Check sheet for the modelled part. Datum: model origin and axes. Units: mm. Face numbers are marked on the shaded views. A direction names the side the tool comes from. Give positions to 0.01 mm unless a question says otherwise; leave off trailing zeros. Order: outer loops, then holes, each group sorted by start corner. A loop starts at its lowest first (then second) coordinate and runs counter-clockwise, first axis right, second up.
```python
from build123d import *

# Parameters (mm, degrees)
F0_R     = 3.175
F1_DEPTH = 19.05
F2_R     = 3.175
F3_DEPTH = 25.4
F4_R     = 6.35


with BuildPart() as f1:
    # F0 (on Top) → F1 (new body)
    with BuildSketch(Plane.XY):
        Polygon((21.1725122346, -375.6896027952), (21.1725122346, -220.1146027952), (10.0600122346, -220.1146027952), (10.0600122346, -188.3646027952), (-15.3399877654, -188.3646027952), (-15.3399877654, -210.5896027952), (-15.3399877654, -220.1146027952), (-26.4524877654, -220.1146027952), (-26.4524877654, -248.6896067858), (-47.0899877654, -248.6896067858), (-47.0899877654, -293.1396027952), (-96.3024877654, -293.1396027952), (-96.3024877654, -314.9836027952), (-96.3024877654, -340.3836027952), (-47.0899877654, -340.3836027952), (-47.0899877654, -375.6896027952), (-26.4524877654, -375.6896027952), (-13.7524877654, -375.6896027952), align=None)
        with Locations((-37.5649877654, -366.1646027952)):
            Circle(F0_R, mode=Mode.SUBTRACT)
        with Locations((-37.5649877654, -258.2146027952)):
            Circle(F0_R, mode=Mode.SUBTRACT)
        with Locations((-2.6399877654, -235.9896027952)):
            Circle(F0_R, mode=Mode.SUBTRACT)
        with Locations((-2.6399877654, -210.5896027952)):
            Circle(F0_R, mode=Mode.SUBTRACT)
    extrude(amount=F1_DEPTH)

    # F2 (on face) → F3 (cut)
    with BuildSketch(Plane.XY.offset(19.05)):
        with Locations((-18.5149877654, -232.8146027952)):
            Circle(F2_R)
        with Locations((13.2350122346, -232.8146027952)):
            Circle(F2_R)
        with Locations((13.2350122346, -258.2146027952)):
            Circle(F2_R)
        with Locations((-18.5149877654, -258.2146027952)):
            Circle(F2_R)
    extrude(amount=-F3_DEPTH, mode=Mode.SUBTRACT)

    # F4
    f4_edges = [f1.edges().sort_by_distance(p)[0] for p in [
        (-96.302488, -340.383603, 9.525),
        (-96.302488, -293.139603, 9.525),
    ]]
    fillet(f4_edges, radius=F4_R)


solid = f1.part
```
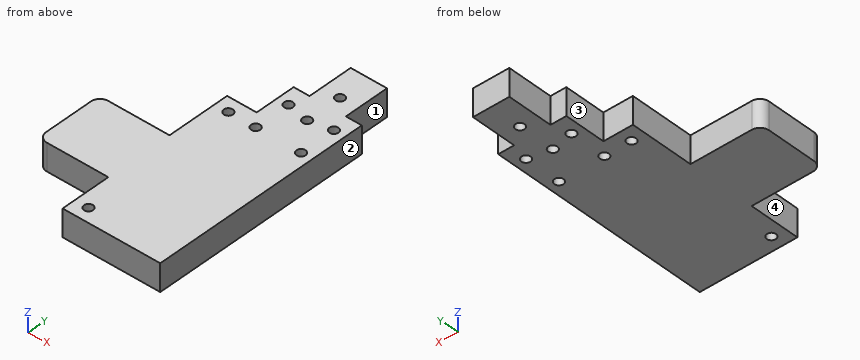
(1) Cross-section at A-A on z = 3. Count the separate pieces of the cut face and the enclosed holes in it, then the cut area to 3 significant figures.
Response values:
separate pieces: 1
enclosed holes: 8
area: 12,900 mm2
(2) Material ranges on L1, parallel to Y at x = -2.5, z = 4; L2, parallel to Y at x = -37.5, z = 5; L3, parallel to X at y = -285, z = 16.75, recorded low to high.
Response values:
L1: y = -375.69 to -239.16, -232.82 to -213.76, -207.42 to -188.36
L2: y = -375.69 to -369.34, -362.99 to -261.39, -255.04 to -248.69
L3: x = -47.09 to 21.17
(3) Cross-section at C-C on y = -346.5. Enter the section's corners in (x, z).
Response values:
outline: (-47.09, 0) - (21.17, 0) - (21.17, 19.05) - (-47.09, 19.05) - close
(4) Gauge pin test, flat ends, axial feed: pin 1 Ø3.5 at (x, z) = (-20, 6) entering from +Y; pin 2 Ø10 at (y, z) = (-287.5, 11) entering from -X; pin 3 Ø9.5 at (x, z) = (-66.5, 10) entering from +Y. Record the tip position at first contact, or that the pin passes through.
Response values:
pin 1: stops at y = -220.11
pin 2: stops at x = -47.09
pin 3: stops at y = -293.14
(5) Cross-section at B-B on x = -70.5. Enter the section's corners in (y, z).
Response values:
outline: (-340.38, 0) - (-293.14, 0) - (-293.14, 19.05) - (-340.38, 19.05) - close
(6) Set-up check for the marked faces 1, 2, 3 and 4: record each of +Z, -Z, +X, -X, +Y, -Y from which the full face is reachable in a straight line by a thin tool's end or side.
Response values:
face 1: +Z, -Z, +X, +Y
face 2: +Z, -Z, +X, +Y, -Y
face 3: +Z, -Z, -X, +Y
face 4: +Z, -Z, -X, -Y
